The listing builds one solid part. Answer for the finished solid, in the listing's coordinates (mm). A direction names the side the tool comes from. Coordinates: 2 decimals unless noted, no trailing zeros. Order: outer loops, then holes, each group sorted by start corner. A loop starts at its lowest first (then second) coordinate and runs counter-clockwise, first axis right, second up. Notation, with made-up numbers: (2.5, 30) -> (30.5, 30) arc R25 cw to (30.5, 60) -> close; hole circle Ø7 at (80.25, 46.5). An arc over 180 degrees is marked (long way). Answer in a Markdown table with one row per item.
```python
from build123d import *

# Parameters (mm, degrees)
F0_W      = 50.8
F0_H      = 31.75
F1_DEPTH  = 6.35
F3_DEPTH  = 25.4
F4_W      = 50.8
F4_H      = 12.7
F5_DEPTH  = 38.1
F6_R      = 3.175
F7_DEPTH  = 25.4
F9_DEPTH  = 25.4
F10_DEPTH = 25.4
F12_DEPTH = 12.7
F14_DEPTH = 12.7
F15_R     = 5.8141785566
F16_DEPTH = 19.05


# Not quite as in the source:
# - a feature names something its author has since deleted; it is built from what else it names


with BuildPart() as f1:
    # F0 (on Top) → F1 (new body)
    with BuildSketch(Plane.XY):
        with Locations((25.4, 15.875)):
            Rectangle(F0_W, F0_H)
    extrude(amount=F1_DEPTH)

    # F2 (on face) → F3 (cut)
    with BuildSketch(Plane.XY.offset(6.35)):
        with BuildLine():
            ThreePointArc((6.35, 0), (1.8598719395, 1.8598719395), (0, 6.35))
            Line((0, 6.35), (0, 0))
            Line((0, 0), (6.35, 0))
        make_face()
        with BuildLine():
            ThreePointArc((50.8, 6.35), (48.9401280605, 1.8598719395), (44.45, 0))
            Line((44.45, 0), (50.8, 0))
            Line((50.8, 0), (50.8, 6.35))
        make_face()
    extrude(amount=-F3_DEPTH, mode=Mode.SUBTRACT)

    # F4 (on face) → F5 (join)
    with BuildSketch(Plane.XY.offset(6.35)):
        with Locations((25.4, 25.4)):
            Rectangle(F4_W, F4_H)
    extrude(amount=F5_DEPTH)

    # F6 (on face) → F7 (cut)
    with BuildSketch(Plane.XY.offset(6.35)):
        with Locations((9.525, 12.7)):
            Circle(F6_R)
        with Locations((41.275, 12.7)):
            Circle(F6_R)
    extrude(amount=-F7_DEPTH, mode=Mode.SUBTRACT)

    # F8 (on face) → F9 (cut)
    with BuildSketch(Plane.XZ.offset(-19.05)):
        with BuildLine():
            Line((12.7, 19.05), (12.7, 44.45))
            Line((12.7, 44.45), (0, 44.45))
            Line((0, 44.45), (0, 6.35))
            ThreePointArc((0, 6.35), (8.9802561211, 10.0697438789), (12.7, 19.05))
        make_face()
        with BuildLine():
            Line((50.8, 44.45), (38.1, 44.45))
            Line((38.1, 44.45), (38.1, 19.05))
            ThreePointArc((38.1, 19.05), (41.8197438789, 10.0697438789), (50.8, 6.35))
            Line((50.8, 6.35), (50.8, 44.45))
        make_face()
    extrude(amount=-F9_DEPTH, mode=Mode.SUBTRACT)

    # F8 (on face) → F10 (cut)
    with BuildSketch(Plane.XZ.offset(-19.05)):
        with BuildLine():
            Line((12.7, 19.05), (12.7, 44.45))
            Line((12.7, 44.45), (0, 44.45))
            Line((0, 44.45), (0, 6.35))
            ThreePointArc((0, 6.35), (8.9802561211, 10.0697438789), (12.7, 19.05))
        make_face()
        with BuildLine():
            Line((38.1, 44.45), (12.7, 44.45))
            ThreePointArc((12.7, 44.45), (25.4, 31.75), (38.1, 44.45))
        make_face()
        with BuildLine():
            Line((50.8, 44.45), (38.1, 44.45))
            Line((38.1, 44.45), (38.1, 19.05))
            ThreePointArc((38.1, 19.05), (41.8197438789, 10.0697438789), (50.8, 6.35))
            Line((50.8, 6.35), (50.8, 44.45))
        make_face()
    extrude(amount=-F10_DEPTH, mode=Mode.SUBTRACT)

    # F11 (on face) → F12 (join)
    with BuildSketch(Plane.XZ.offset(-19.05)):
        with BuildLine():
            ThreePointArc((12.7, 44.45), (25.4, 31.75), (38.1, 44.45))
            ThreePointArc((38.1, 44.45), (25.4, 57.15), (12.7, 44.45))
        make_face()
    extrude(amount=-F12_DEPTH)

    # F13 (on face) → F14 (join)
    with BuildSketch(Plane.XZ.offset(-19.05)):
        with BuildLine():
            ThreePointArc((12.7, 44.45), (25.4, 31.75), (38.1, 44.45))
            ThreePointArc((38.1, 44.45), (25.4, 57.15), (12.7, 44.45))
        make_face()
    extrude(amount=F14_DEPTH)

    # F15 (on face) → F16 (cut)
    with BuildSketch(Plane.XZ.offset(-6.35)):
        with Locations((25.4, 44.45)):
            Circle(F15_R)
    extrude(amount=-F16_DEPTH, mode=Mode.SUBTRACT)


solid = f1.part
```
(1) A cutting plane is placed at C-C, the plane x = 25.4. Determine the outline of the cut face in (y, z).
Check values:
| item | result |
|---|---|
| outline | (0, 0) -> (31.75, 0) -> (31.75, 57.15) -> (6.35, 57.15) -> (6.35, 50.26) -> (25.4, 50.26) -> (25.4, 38.64) -> (6.35, 38.64) -> (6.35, 31.75) -> (19.05, 31.75) -> (19.05, 6.35) -> (0, 6.35) -> close |
(2) For a pull along X with two mould halves and no side action, classify faces 1 (the flat face through (31, 6.35, 42)), 2 (the flat face through (38.1, 25, 32)), 3 (the cylindrical face through (38.1, 12.8, 3.2)) as released by +X, released by -X, zero draft, split by the parting line, or undercut.
Check values:
| item | result |
|---|---|
| face 1 | zero draft |
| face 2 | released by +X |
| face 3 | undercut |
(3) A cutting plane is placed at A-A, the plane y = 12.7. Determine the outline of the cut face in (x, z).
Check values:
| item | result |
|---|---|
| outline | (0, 0) -> (6.35, 0) -> (6.35, 6.35) -> (0, 6.35) -> close; (12.7, 0) -> (38.1, 0) -> (38.1, 6.35) -> (12.7, 6.35) -> close; circle Ø25.4 at (25.4, 44.45); (44.45, 0) -> (50.8, 0) -> (50.8, 6.35) -> (44.45, 6.35) -> close; hole circle Ø11.63 at (25.4, 44.45) |
(4) A cutting plane is placed at B-B, the plane y = 17. Determine the outline of the cut face in (x, z).
Check values:
| item | result |
|---|---|
| outline | (0, 0) -> (50.8, 0) -> (50.8, 6.35) -> (0, 6.35) -> close; circle Ø25.4 at (25.4, 44.45); hole circle Ø11.63 at (25.4, 44.45) |
(5) A cutting plane is placed at D-D, the plane z = 37. Determine the outline of the cut face in (x, y).
Check values:
| item | result |
|---|---|
| outline | (12.7, 19.05) -> (15.11, 19.05) -> (15.11, 6.35) -> (35.69, 6.35) -> (35.69, 19.05) -> (38.1, 19.05) -> (38.1, 31.75) -> (12.7, 31.75) -> close |
(6) Find the intervals of material crossed by line 1 along Z through (x, y) = (25, 16); line 2 along Z through (x, y) = (25.4, 16.25); line 3 along X through (y, z) = (19, 40), in increasing order. Write a range as from..to.
Check values:
| item | result |
|---|---|
| line 1 | 0..6.35, 31.76..38.65, 50.25..57.14 |
| line 2 | 0..6.35, 31.75..38.64, 50.26..57.15 |
| line 3 | 13.51..21.66, 29.14..37.29 |
(7) Flat-ended cylindrical pins translate along their axes: pin 1 (2 mm diameter, centred on x = 29.5, y = 20, fed in from -Z); pin 2 (4 mm diameter, centred on y = 27, z = 19.5, fed in from -X); pin 3 (3.5 mm diameter, centred on x = 23, z = 45, fed in from -Y); pin 4 (6.5 mm diameter, centred on y = 28.5, z = 27, fed in from -X). Find the tip coordinate at first contact, or state that the pin passes through.
Check values:
| item | result |
|---|---|
| pin 1 | z = 0 |
| pin 2 | x = 12.61 |
| pin 3 | y = 25.4 |
| pin 4 | x = 12.7 |
(8) Which of the six approach directions +Z, -Z, +X, -X, +Y, -Y give full straight-line access (tool end or side, diameter ignored) to faces 4 (the cylindrical face through (28.53, 15.74, 49.35)), 5 (the flat face through (25, 10, 6.35)), 6 (the flat face through (12.7, 25, 32)), 7 (the flat face through (25, 16, 0)), 8 (the flat face through (25, 31.75, 23))?
Check values:
| item | result |
|---|---|
| face 4 | -Y |
| face 5 | +X, -X, -Y |
| face 6 | +Z, -X, +Y, -Y |
| face 7 | -Z, +X, -X, +Y, -Y |
| face 8 | +Z, -Z, +X, -X, +Y |
